```python
from build123d import *

# Parameters (mm, degrees)
F1_DEPTH = 63.5
F2_R     = 152.4
F3_R     = 5.08
F4_R     = 5.08


with BuildPart() as f1:
    # F0 (on Top) → F1 (new body)
    with BuildSketch(Plane.XY):
        with BuildLine():
            Line((139.7, -6.35), (266.7, -6.35))
            Line((266.7, -6.35), (266.7, 6.35))
            Line((266.7, 6.35), (145.47977, 6.35))
            ThreePointArc((145.47977, 6.35), (130.864429, 7.052433), (116.383816, 9.153257))
            ThreePointArc((116.383816, 9.153257), (0, 20.366286), (-116.383816, 9.153257))
            ThreePointArc((-116.383816, 9.153257), (-130.864429, 7.052433), (-145.47977, 6.35))
            Line((-145.47977, 6.35), (-266.7, 6.35))
            Line((-266.7, 6.35), (-266.7, -6.35))
            Line((-266.7, -6.35), (-139.7, -6.35))
            ThreePointArc((-139.7, -6.35), (0, 9.873164), (139.7, -6.35))
        make_face()
    extrude(amount=F1_DEPTH)

    # F2
    f2_edges = [f1.edges().sort_by_distance(p)[0] for p in [
        (139.7, -6.35, 31.75),
        (-139.7, -6.35, 31.75),
    ]]
    fillet(f2_edges, radius=F2_R)

    # F3
    f3_edges = [f1.edges().sort_by_distance(p)[0] for p in [
        (-211.54992, -6.35, 63.5),
        (-206.089885, 6.35, 63.5),
    ]]
    fillet(f3_edges, radius=F3_R)

    # F4
    f4_edges = [f1.edges().sort_by_distance(p)[0] for p in [
        (-206.089885, 6.35, 0),
        (-211.54992, -6.35, 0),
    ]]
    fillet(f4_edges, radius=F4_R)


solid = f1.part
```
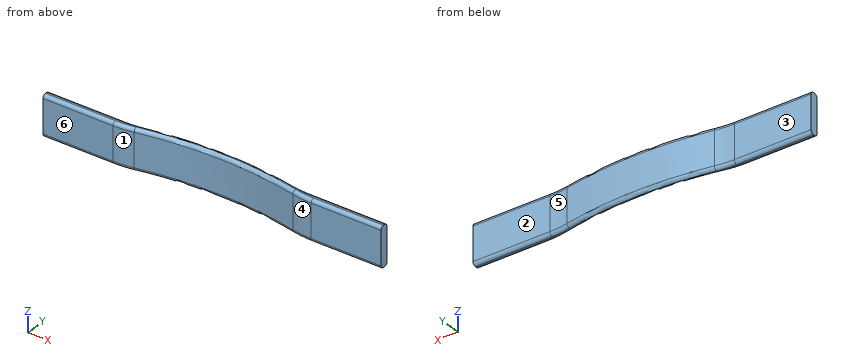
Could you check a few things on this model? Use its own coordinates, in mm. Face numbers are marked on the shaded views. A direction names the side the tool comes from. Round coordinates to 2 decimals unless told otherwise and drop trailing zeros. Loops run counter-clockwise (first coordinate to the right, second up) from the corner with the lowest first, then second, coordinate; pieces in that order, holes last. Notation, with made-up numbers: (69.5, 28) - (77.5, 28) arc R9 cw to (77.5, 33) - close; hole circle Ø4 at (52.5, 58.25). An arc over 180 degrees is marked (long way). Answer in a Markdown table with one row per item. Add a question column.
(1) If we section it at B-B (x = 223.5): Please give me the cut outline in (y, z).
(2) If we mould it in two halves opening along X, with no side actions, what happens to the marked faces 4, 5 and 6? For each: pulls with the +X half, pulls with the -X half, needs draft (parallel to the pull), parting line crosses it, or undercut.
(3) For the marked faces 1, 2 and 3, which set-ups out of +Z, -Z, +X, -X, +Y, -Y let a thin tool reach every point of the face, with its end or its side?
(4) I'm going to push flat-ended pins straight in: pin 1 (3 mm diameter, centred on x = -136, z = 40, fed in from -Y); pin 2 (4 mm diameter, centred on x = 132, y = -2, fed in from +Z); pin 3 (1 mm diameter, centred on x = -186.5, z = 20.5, fed in from +Y). Where does each tip first touch, or does it pass through?
(5) If we section it at A-A (z = 28): Please give me the cut outline in (x, y), plus the area to 4 significant figures.
(6) I need wall thicknesses on line 1 along Y through (x, z) = (-187, 36.5); line 2 along Z through (x, y) = (-74.5, 6). Which ranges of each line are inside material? Lowest first, please.
Model answer:
| question | item | result |
|---|---|---|
| 1 | outline | (-6.35, 5.08) arc R5.08 ccw to (-1.27, 0) - (1.27, 0) arc R5.08 ccw to (6.35, 5.08) - (6.35, 58.42) arc R5.08 ccw to (1.27, 63.5) - (-1.27, 63.5) arc R5.08 ccw to (-6.35, 58.42) - close |
| 2 | face 4 | undercut |
| 2 | face 5 | pulls with the +X half |
| 2 | face 6 | needs draft |
| 3 | face 1 | +Z, -Z, -Y |
| 3 | face 2 | +Z, -Z, +X, +Y |
| 3 | face 3 | +Z, -Z, -X, +Y |
| 4 | pin 1 | stops at y = -5.17 |
| 4 | pin 2 | stops at z = 63.45 |
| 4 | pin 3 | stops at y = 6.35 |
| 5 | outline | (-266.7, -6.35) - (-156.4, -6.35) arc R152.4 ccw to (-125.12, -3.11) arc R609.6 cw to (125.12, -3.11) arc R152.4 ccw to (156.4, -6.35) - (266.7, -6.35) - (266.7, 6.35) - (145.48, 6.35) arc R152.4 cw to (116.38, 9.15) arc R609.6 ccw to (-116.38, 9.15) arc R152.4 cw to (-145.48, 6.35) - (-266.7, 6.35) - close |
| 5 | area | 6,175 mm² |
| 6 | line 1 | y = -6.35 to 6.35 |
| 6 | line 2 | z = 2.52 to 60.98 |
